Autodesk Inventor part; units mm, degrees
ref_plane "YZ Plane" through (0, 0, 0) normal (1, 0, 0) x (0, 1, 0)
ref_plane "XZ Plane" through (0, 0, 0) normal (0, 1, 0) x (-1, 0, 0)
ref_plane "XY Plane" through (0, 0, 0) normal (0, 0, 1) x (1, 0, 0)
sketch "Sketch1" plane through (0, 0, 0) normal (0, 0, 1) x (1, 0, 0)
  circle A0 centre (-4.8387, 12.596) radius 18.2563
  dimension "d0" = 36.5125
extrude "Extrusion1" add sketch "Sketch1" along normal blind 203.2
chamfer "Chamfer1" distance 3.9688 distance2 25.4 1 edges at (-23.095, 12.596, 0) measured on face at (1.1407, 16.9825, 0)
chamfer "Chamfer2" distance 25.4 distance2 3.9688 1 edges at (-23.095, 12.596, 203.2) measured on face at (13.1811, 9.6675, 143.9333)
properties part number "FE-00001-04"
Check sheet for the modelled part. Datum: model origin and axes. Units: mm. Coordinates: 2 decimals unless noted, no trailing zeros. Loops run counter-clockwise (first coordinate to the right, second up) from the corner with the lowest first, then second, coordinate; pieces in that order, holes last.
1) Sectioned sample at B-B (z = 91). Record the boundary of the cut face in (x, y), and give its area (3 significant figures).
2) Release check for a two-part mould opening along Z. For faces 1 (the face through (10.288, 7.832, 193.144)), 2 (the face through (-5, 13, 0)), 3 (the face through (-7.215, -5.505, 100.533)) record: released by +Z, released by -Z, zero draft, split by the parting line, or undercut.
3) Gauge pin test, flat ends, axial feed: pin 1 (10 mm diameter, centred on x = -13, z = 64, fed in from -Y); pin 2 (3 mm diameter, centred on y = 18.5, z = 126, fed in from +X); pin 3 (4 mm diameter, centred on y = 20.5, z = 31, fed in from +X). Record the tip position at first contact, or that the pin passes through.
4) Sectioned sample at A-A (z = 183). Record the boundary of the cut face in (x, y), and give its area (3 significant figures).
5) Material ranges on probe 1 along Y at (x, z) = (-5, 42.5); probe 2 along Y at (x, z) = (6.5, 158); probe 3 along X at (y, z) = (14, 107.5), recorded low to high.
Check sheet entries:
1. outline: circle Ø36.51 at (-4.84, 12.6)
1. area: 1,050 mm2
2. face 1: released by +Z
2. face 2: released by -Z
2. face 3: zero draft
3. pin 1: stops at y = -5.38
3. pin 2: stops at x = 12.88
3. pin 3: stops at x = 12.44
4. outline: circle Ø34.89 at (-4.84, 12.6)
4. area: 956 mm2
5. probe 1: y = -5.66 to 30.85
5. probe 2: y = -1.71 to 26.9
5. probe 3: x = -23.04 to 13.36
